Input: part model. Units: mm. Frame: model coordinates. Round coordinates to 2 decimals unless told otherwise and drop trailing zeros. Loops run counter-clockwise (first coordinate to the right, second up) from the corner with the lowest first, then second, coordinate; pieces in that order, holes last.
1) Section D-D, the plane x = -106.5. Return loops of the section in (y, z), and give its area (4 significant figures).
2) Section C-C, the plane y = 1.45. State how many separate pieces and enclosed holes the cut face has, and give its area (3 significant figures).
3) Ray query, line 1 along Z through (x, y) = (-148, 0.65); line 2 along Z through (x, y) = (-104, 0.8); line 3 along X through (y, z) = (0.35, -12.5). Return the intervals inside material, ascending.
4) Draft query along Z for faces 1 (the face through (-125, 0, 10)), 2 (the face through (-152.994, 0.986, 2.038)). Return one class per face: pulls with the +Z half, pulls with the -Z half, needs draft (parallel to the pull), parting line crosses it, or undercut.
5) First-contact query: pin 1 (12 mm diameter, centred on x = -123.16, z = -14.98, fed in from -Y); pin 2 (6 mm diameter, centred on x = -139.66, z = 0.02, fed in from +Y). Flat tips, straight axial feed; report the tip coordinate or a pass-through.
6) Section A-A, the plane x = -151. Return loops of the section in (y, z), and give its area (3 significant figures).
7) Section B-B, the plane z = 14. Return loops of the section in (x, y).
from build123d import *

# Parameters (mm, degrees)
SKETCH2_W           = 140
SKETCH2_H           = 83
SKETCH2_R           = 3.75
SKETCH2_R_2         = 3.5
SKETCH2_W_2         = 45.5
SKETCH2_H_2         = 26
SKETCH2_W_3         = 12.5
SKETCH2_H_3         = 5.3
BOSS_EXTRUDE1_DEPTH = 2
CHAMFER1_SIZE       = 1


with BuildPart() as part:
    # Sketch2 → Boss-Extrude1 (new body)
    with BuildSketch(Plane(origin=(0, 0, 0), x_dir=(1, 0, 0), z_dir=(0, 1, 0))):
        with Locations((-123.656387665, -10.354625551)):
            Rectangle(SKETCH2_W, SKETCH2_H)
        with Locations(Location((-156.156387665, 14.977524107, 0), (0, 0, 270))):
            Circle(SKETCH2_R, mode=Mode.SUBTRACT)
        with Locations(Location((-139.656387665, 14.977524107, 0), (0, 0, 270))):
            Circle(SKETCH2_R, mode=Mode.SUBTRACT)
        with Locations(Location((-123.156387665, 14.977524107, 0), (0, 0, 270))):
            Circle(SKETCH2_R, mode=Mode.SUBTRACT)
        with Locations(Location((-123.156387665, -0.022475893, 0), (0, 0, 270))):
            Circle(SKETCH2_R, mode=Mode.SUBTRACT)
        with Locations(Location((-139.656387665, -0.022475893, 0), (0, 0, 270))):
            Circle(SKETCH2_R, mode=Mode.SUBTRACT)
        with Locations(Location((-156.156387665, -0.022475893, 0), (0, 0, 270))):
            Circle(SKETCH2_R, mode=Mode.SUBTRACT)
        with Locations(Location((-85.656387665, 1.339603921, 0), (0, 0, 270))):
            Circle(SKETCH2_R_2, mode=Mode.SUBTRACT)
        with Locations(Location((-104.656387665, 1.339603921, 0), (0, 0, 270))):
            Circle(SKETCH2_R_2, mode=Mode.SUBTRACT)
        with Locations((-139.906387665, -25.354625551)):
            Rectangle(SKETCH2_W_2, SKETCH2_H_2, mode=Mode.SUBTRACT)
        with Locations((-104.906387665, -15.00079349)):
            Rectangle(SKETCH2_W_3, SKETCH2_H_3, mode=Mode.SUBTRACT)
    extrude(amount=BOSS_EXTRUDE1_DEPTH)

    # Chamfer1
    chamfer1_edges = [part.edges().sort_by_distance(p)[0] for p in [
        (-193.656387665, 2, 10.354625551),
        (-123.656387665, 2, 51.854625551),
        (-53.656387665, 2, 10.354625551),
        (-123.656387665, 2, -31.145374449),
    ]]
    chamfer(chamfer1_edges, length=CHAMFER1_SIZE)


solid = part.part
Final values:
1. outline: (0, -31.15) - (1, -31.15) - (2, -30.15) - (2, -4.31) - (0, -4.31) - close; (0, 1.64) - (2, 1.64) - (2, 12.35) - (0, 12.35) - close; (0, 17.65) - (2, 17.65) - (2, 50.85) - (1, 51.85) - (0, 51.85) - close
1. area: 142.5 mm2
2. separate pieces: 1
2. enclosed holes: 10
2. area: 9,830 mm2
3. line 1: z = -31.15 to 12.35, 38.35 to 51.85
3. line 2: z = -31.15 to -4.78, 2.1 to 12.35, 17.65 to 51.85
3. line 3: x = -193.66 to -158.97, -153.34 to -142.47, -136.84 to -125.97, -120.34 to -53.66
4. face 1: needs draft
4. face 2: undercut
5. pin 1: stops at y = 0
5. pin 2: passes through
6. outline: (0, -31.15) - (1, -31.15) - (2, -30.15) - (2, 12.35) - (0, 12.35) - close; (0, 38.35) - (2, 38.35) - (2, 50.85) - (1, 51.85) - (0, 51.85) - close
6. area: 113 mm2
7. outline: (-193.66, 0) - (-162.66, 0) - (-162.66, 2) - (-192.66, 2) - (-193.66, 1) - close; (-117.16, 0) - (-111.16, 0) - (-111.16, 2) - (-117.16, 2) - close; (-98.66, 0) - (-53.66, 0) - (-53.66, 1) - (-54.66, 2) - (-98.66, 2) - close
